The listing builds one solid part. Answer for the finished solid, in the listing's coordinates (mm). A direction names the side the tool comes from. Give positions to 0.01 mm unless a question says otherwise; leave off trailing zeros. Write each loop counter-clockwise with the first axis right and the second up, starting at its lowest first coordinate (ties: lowest second). Pieces come first, ordered by that corner, then holes. Notation, with made-up numbers: (38.25, 42.25) - (78.25, 42.25) arc R15 cw to (78.25, 65.25) - close; hole circle Ø4 at (-16.5, 22.5). An arc over 180 degrees is marked (long way). Return JSON: item names as keys, results as strings.
from build123d import *

# Parameters (mm, degrees)
F0_R          = 10
F1_DEPTH      = 30
F2_R          = 2.85
F3_DEPTH      = 15
F4_R          = 3.5
F5_DEPTH      = 10
F5_DEPTH_BACK = 10
F7_W          = 11.9265963338
F7_H          = 6
F8_DEPTH      = 10
F8_DEPTH_BACK = 10
F9_SIZE       = 1.5


with BuildPart() as f1:
    # F0 (on Top) → F1 (new body)
    with BuildSketch(Plane.XY):
        Circle(F0_R)
    extrude(amount=-F1_DEPTH)

    # F2 (on face) → F3 (cut)
    with BuildSketch(Plane.XY):
        Circle(F2_R)
    extrude(amount=-F3_DEPTH, mode=Mode.SUBTRACT)

    # F4 (on Right) → F5 (cut, two sides)
    with BuildSketch(Plane.YZ) as f5_sk:
        with Locations((0, -22.625)):
            Circle(F4_R)
    extrude(amount=-F5_DEPTH, mode=Mode.SUBTRACT)
    extrude(f5_sk.sketch, amount=F5_DEPTH_BACK, mode=Mode.SUBTRACT)

    # F7 (on Right) → F8 (cut, two sides)
    with BuildSketch(Plane.YZ) as f8_sk:
        with Locations((-5.9632981669, -22.625)):
            Rectangle(F7_W, F7_H)
    extrude(amount=-F8_DEPTH, mode=Mode.SUBTRACT)
    extrude(f8_sk.sketch, amount=F8_DEPTH_BACK, mode=Mode.SUBTRACT)

    # F9
    f9_edges = [f1.edges().sort_by_distance(p)[0] for p in [
        (-2.85, 0, 0),
        (-10, 0, 0),
        (-10, 0, -30),
    ]]
    chamfer(f9_edges, length=F9_SIZE)


solid = f1.part
Item 1: Consider L1, parallel to Z at x = -1.5, y = -7.5 (3 decimals); L2, parallel to Y at x = 0, z = -6.25; L3, parallel to Z at x = 1.5, y = 0 (3 decimals). Determine where each line is inside the solid, lowest interval first.
Answer below:
{"L1": "z = -30 to -25.625, -19.625 to 0", "L2": "y = -10 to -2.85, 2.85 to 10", "L3": "z = -30 to -26.125, -19.125 to -15"}
Item 2: The mould has two halves that part along Z. Classify faces 1 (the face through (0, 0, -30)), 2 (the face through (0, 0, -15)), 3 (the face through (0, -5, -19.625)): +Z half, -Z half, draft (parallel to the pull), parting line (faces both ways), or undercut.
Answer below:
{"face 1": "-Z half", "face 2": "+Z half", "face 3": "undercut"}
Item 3: A cutting plane is placed at C-C on z = -3.5. Determine the outline of the cut face in (x, y).
Answer below:
{"outline": "circle Ø20 at (0, 0); hole circle Ø5.7 at (0, 0)"}
Item 4: A cutting plane is placed at B-B on x = 0. Determine the outline of the cut face in (y, z) (3 decimals), then the cut area to 3 significant figures.
Answer below:
{"outline": "(-10, -28.5) - (-8.5, -30) - (8.5, -30) - (10, -28.5) - (10, -1.5) - (8.5, 0) - (4.35, 0) - (2.85, -1.5) - (2.85, -15) - (-2.85, -15) - (-2.85, -1.5) - (-4.35, 0) - (-8.5, 0) - (-10, -1.5) - (-10, -19.625) - (-1.803, -19.625) arc R3.5 cw (long way) to (-1.803, -25.625) - (-10, -25.625) - close", "area": "427 mm²"}
Item 5: A cutting plane is placed at A-A on y = 0. Determine the outline of the cut face in (x, z) (3 decimals).
Answer below:
{"outline": "(-10, -28.5) - (-8.5, -30) - (8.5, -30) - (10, -28.5) - (10, -26.125) - (-10, -26.125) - close; (-10, -19.125) - (10, -19.125) - (10, -1.5) - (8.5, 0) - (4.35, 0) - (2.85, -1.5) - (2.85, -15) - (-2.85, -15) - (-2.85, -1.5) - (-4.35, 0) - (-8.5, 0) - (-10, -1.5) - close"}
Item 6: For faces 4 (the face through (0, -5, -25.625)), 5 (the face through (-0.1, 3.5, -22.7)), 6 (the face through (-2.262, -1.734, -8.156)), determine the directions among +Z, -Z, +X, -X, +Y, -Y from which every point of the face is accessible in a straight line to the end or side of a thin tool.
Answer below:
{"face 4": "+X, -X, -Y", "face 5": "+X, -X", "face 6": "+Z"}
Item 7: A cutting plane is placed at D-D on z = -17.75. Determine the outline of the cut face in (x, y).
Answer below:
{"outline": "circle Ø20 at (0, 0)"}
Item 8: Flat-ended cylindrical pins translate along their axes: P1, Ø2, axis at x = -1.5, y = 2, coming from the +Z side; P2, Ø4, axis at y = -7, z = -16, coming from the -X side; P3, Ø3, axis at x = -0.5, y = 1.5, coming from the +Z side; P4, Ø1.5, axis at y = 0.5, z = -22, coming from the -X side. Find the tip coordinate at first contact, or state that the pin passes through.
Answer below:
{"P1": "stops at z = -0.85", "P2": "stops at x = -8.66", "P3": "stops at z = -1.27", "P4": "passes through"}
